Geometry: final body of the model. Coordinates: model frame, mm. Face numbers are marked on the shaded views. A direction names the side the tool comes from. Coordinates: 2 decimals unless noted, no trailing zeros. Loops run counter-clockwise (first coordinate to the right, second up) from the corner with the lowest first, then second, coordinate; pieces in that order, holes last. Notation, with made-up numbers: (-12, 61.25) - (2, 61.25) arc R12 cw to (2, 84.25) - close; hole circle Ø8 at (-12, 34.5). An arc over 180 degrees is marked (long way). Return JSON: item names as keys, results as strings.
from build123d import *

# Parameters (mm, degrees)
BOSS_EXTRUDE1_DEPTH = 23
SKETCH2_R           = 2.5
BOSS_EXTRUDE2_DEPTH = 1.5
SKETCH3_R           = 0.5
BOSS_EXTRUDE3_DEPTH = 7
FILLET1_R           = 1
FILLET2_R           = 3
BOSS_EXTRUDE4_DEPTH = 1
FILLET3_R           = 0.5


with BuildPart() as part:
    # Sketch1 → Boss-Extrude1 (new body)
    with BuildSketch(Plane.XY):
        with BuildLine():
            Line((-6.614378278, 7.5), (6.614378278, 7.5))
            ThreePointArc((6.614378278, 7.5), (10, 0), (6.614378278, -7.5))
            Line((6.614378278, -7.5), (-6.614378278, -7.5))
            ThreePointArc((-6.614378278, -7.5), (-10, 0), (-6.614378278, 7.5))
        make_face()
    extrude(amount=BOSS_EXTRUDE1_DEPTH)

    # Sketch2 → Boss-Extrude2 (add)
    with BuildSketch(Plane.XY.offset(23)):
        Circle(SKETCH2_R)
    extrude(amount=BOSS_EXTRUDE2_DEPTH)

    # Sketch3 → Boss-Extrude3 (add)
    with BuildSketch(Plane.XY.offset(24.5)):
        Circle(SKETCH3_R)
    extrude(amount=BOSS_EXTRUDE3_DEPTH)

    # Fillet1
    fillet1_edges = [part.edges().sort_by_distance(p)[0] for p in [
        (10, 0, 23),
        (0, 7.5, 23),
        (-10, 0, 23),
        (0, -7.5, 23),
    ]]
    fillet(fillet1_edges, radius=FILLET1_R)

    # Fillet2
    # the kernel refuses this fillet: 3 mm, written as the material it takes off along each edge
    with BuildSketch(Plane(origin=(-14.114378278, 7.5, 0), x_dir=(0, 0, 1), z_dir=(1, 0, 0))) as fillet2_piece_1:
        with BuildLine():
            CenterArc((FILLET2_R, FILLET2_R), FILLET2_R, 180, 90)
            Line((0, FILLET2_R), (0, 0))
            Line((0, 0), (FILLET2_R, 0))
        make_face()
    extrude(amount=28.228756555, mode=Mode.SUBTRACT)
    with BuildSketch(Plane(origin=(0, 0, 0), x_dir=(-0.027613533277189895, 0.9996186736850955, 0), z_dir=(-0.9996186736850955, -0.027613533277189895, 0))) as fillet2_piece_2:
        with BuildLine():
            CenterArc((10 - FILLET2_R, -FILLET2_R), FILLET2_R, 0, 90)
            Line((10, -FILLET2_R), (10, 0))
            Line((10, 0), (10 - FILLET2_R, 0))
        make_face()
    revolve(axis=Axis((0, 0, 0), (0, 0, -1)), revolution_arc=183.164680097, mode=Mode.SUBTRACT)
    with BuildSketch(Plane(origin=(14.114378278, -7.5, 0), x_dir=(0, 1, 0), z_dir=(-1, 0, 0))) as fillet2_piece_3:
        with BuildLine():
            CenterArc((FILLET2_R, -FILLET2_R), FILLET2_R, 90, 90)
            Line((0, -FILLET2_R), (0, 0))
            Line((0, 0), (FILLET2_R, 0))
        make_face()
    extrude(amount=28.228756555, mode=Mode.SUBTRACT)
    with BuildSketch(Plane(origin=(0, 0, 0), x_dir=(0.02761353327718998, -0.9996186736850955, 0), z_dir=(0.9996186736850955, 0.02761353327718998, 0))) as fillet2_piece_4:
        with BuildLine():
            CenterArc((10 - FILLET2_R, -FILLET2_R), FILLET2_R, 0, 90)
            Line((10 - FILLET2_R, 0), (10, 0))
            Line((10, 0), (10, -FILLET2_R))
        make_face()
    revolve(axis=Axis((0, 0, 0), (0, 0, -1)), revolution_arc=183.164680097, mode=Mode.SUBTRACT)

    # Sketch4 → Boss-Extrude4 (add)
    with BuildSketch(Plane(origin=(0, 0, 0), x_dir=(-1, 0, 0), z_dir=(0, 0, -1))):
        with BuildLine():
            Line((-2.758585466, 1.606625472), (2.758585466, 1.606625472))
            ThreePointArc((2.758585466, 1.606625472), (0, -3.192340705), (-2.758585466, 1.606625472))
        make_face()
    extrude(amount=BOSS_EXTRUDE4_DEPTH)

    # Fillet3
    fillet3_edges = [part.edges().sort_by_distance(p)[0] for p in [
        (0, -3.192340705, -1),
        (0, 1.606625472, -1),
    ]]
    fillet(fillet3_edges, radius=FILLET3_R)


solid = part.part
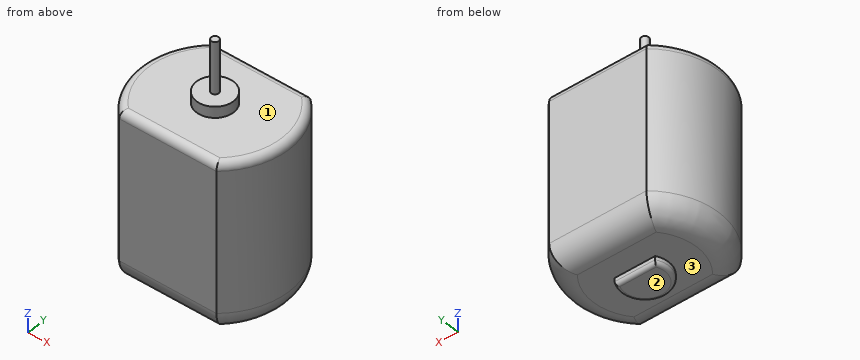
Item 1: First-contact query: pin 1 Ø6 at (y, z) = (4.5, 18) entering from -X; pin 2 Ø1.5 at (x, y) = (-1, -1) entering from +Z; pin 3 Ø1.5 at (y, z) = (5, 13) entering from +X. Flat tips, straight axial feed; report the tip coordinate or a pass-through.
Worked out:
{"pin 1": "x = -9.89", "pin 2": "z = 24.5", "pin 3": "x = 9.05"}
Item 2: Ray query, probe 1 along X at (y, z) = (0, 8); probe 2 along Y at (x, z) = (7.5, 5); probe 3 along Z at (x, y) = (0.5, -1). Return the intervals inside material, ascending. Write a range as from..to.
Worked out:
{"probe 1": "-10..10", "probe 2": "-6.61..6.61", "probe 3": "-1..24.5"}
Item 3: Section query B-B, the plane z = 9. Return loops of the section in (x, y), and give its area (3 significant figures).
Worked out:
{"outline": "(-6.61, -7.5) - (6.61, -7.5) arc R10 ccw to (6.61, 7.5) - (-6.61, 7.5) arc R10 ccw to start", "area": "269 mm^2"}
Item 4: Section query A-A, the plane x = 0. Return loops of the section in (y, z), and give its area (3 significant figures).
Worked out:
{"outline": "(-7.5, 3) arc R3 ccw to (-4.5, 0) - (-3.19, 0) - (-3.19, -0.5) arc R0.5 ccw to (-2.69, -1) - (1.11, -1) arc R0.5 ccw to (1.61, -0.5) - (1.61, 0) - (4.5, 0) arc R3 ccw to (7.5, 3) - (7.5, 22) arc R1 ccw to (6.5, 23) - (2.5, 23) - (2.5, 24.5) - (0.5, 24.5) - (0.5, 31.5) - (-0.5, 31.5) - (-0.5, 24.5) - (-2.5, 24.5) - (-2.5, 23) - (-6.5, 23) arc R1 ccw to (-7.5, 22) - close", "area": "360 mm^2"}
Item 5: Reachability of the marked faces 1, 2 and 3 from +Z, -Z, +X, -X, +Y, -Y: full face, straight path, thin tool, end or side. Return the list, or none.
Worked out:
{"face 1": "+Z", "face 2": "-Z, +X, -X, +Y, -Y", "face 3": "-Z"}
Item 6: Section query C-C, the plane z = 26. Return loops of the section in (x, y).
Worked out:
{"outline": "circle Ø1 at (0, 0)"}
